Can you work these out from the model? Positions are in its coordinate system, mm. Face numbers are marked on the shaded views. A direction names the side the tool comes from. Round coordinates to 2 decimals unless told otherwise and drop trailing zeros. Loops run counter-clockwise (first coordinate to the right, second up) from the corner with the lowest first, then second, coordinate; pieces in that order, holes last. Notation, with made-up numbers: (85, 81) -> (125, 81) arc R27 cw to (125, 102) -> close; hole circle Ø11 at (-4.5, 69). An arc over 180 degrees is marked (long way). Answer as a JSON object with one key per item and string values.
```python
from build123d import *

# Parameters (mm, degrees)
SKETCH1_W           = 32
SKETCH1_H           = 32
BOSS_EXTRUDE1_DEPTH = 30
FILLET1_R           = 6
SKETCH2_R           = 1.5
BOSS_EXTRUDE2_DEPTH = 2.8


with BuildPart() as part:
    # Sketch1 → Boss-Extrude1 (new body)
    with BuildSketch(Plane(origin=(24, 0, 0), x_dir=(0, 0, -1), z_dir=(1, 0, 0))):
        Rectangle(SKETCH1_W, SKETCH1_H)
    extrude(amount=BOSS_EXTRUDE1_DEPTH)

    # Fillet1
    fillet1_edges = [part.edges().sort_by_distance(p)[0] for p in [
        (54, 0, -16),
        (54, 16, 0),
        (54, 0, 16),
        (24, 16, 0),
        (24, 0, -16),
        (24, -16, 0),
        (24, 0, 16),
        (39, 16, 16),
        (39, 16, -16),
        (39, -16, -16),
        (39, -16, 16),
        (54, -16, 0),
    ]]
    fillet(fillet1_edges, radius=FILLET1_R)

    # Sketch2 → Boss-Extrude2 (add)
    with BuildSketch(Plane(origin=(21.2, 0, 0), x_dir=(0, 0, -1), z_dir=(1, 0, 0))):
        with Locations((-4, -4)):
            Circle(SKETCH2_R)
        with Locations((4, -4)):
            Circle(SKETCH2_R)
        with Locations((-4, 4)):
            Circle(SKETCH2_R)
        with Locations((4, 4)):
            Circle(SKETCH2_R)
    extrude(amount=BOSS_EXTRUDE2_DEPTH)


solid = part.part
```
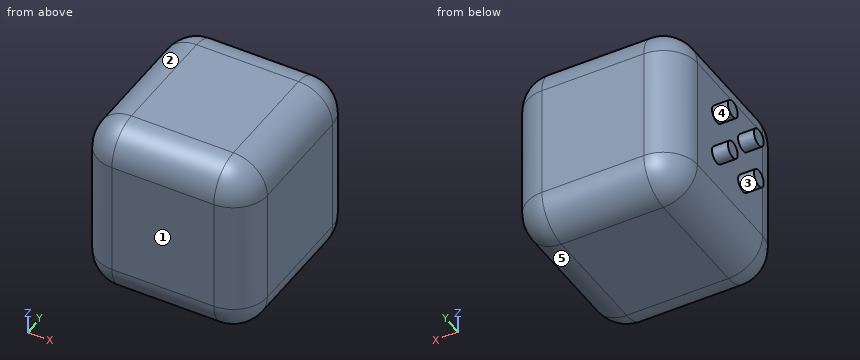
Q1. On a 3-axis mill with a long thin cutter (end or side, diameter ignored), from which of +Z, -Z, +X, -X, +Y, -Y can I reach the whole of each face in a straight line? I mean the marked faces 4 and 5. Say none if no direction works.
Determined:
{"face 4": "-X", "face 5": "-Z, +X, +Y, -Y"}
Q2. I want a section at D-D, the plane z = -9.5. Write out the boundary of the cut face in (x, y).
Determined:
{"outline": "(24, -10) arc R6 ccw to (30, -16) -> (48, -16) arc R6 ccw to (54, -10) -> (54, 10) arc R6 ccw to (48, 16) -> (30, 16) arc R6 ccw to (24, 10) -> close"}
Q3. I want a section at A-A, the plane y = 4. Write out the boundary of the cut face in (x, z), then the cut area to 3 significant figures.
Determined:
{"outline": "(21.2, -5.5) -> (24, -5.5) -> (24, -10) arc R6 ccw to (30, -16) -> (48, -16) arc R6 ccw to (54, -10) -> (54, 10) arc R6 ccw to (48, 16) -> (30, 16) arc R6 ccw to (24, 10) -> (24, 5.5) -> (21.2, 5.5) -> (21.2, 2.5) -> (24, 2.5) -> (24, -2.5) -> (21.2, -2.5) -> close", "area": "946 mm²"}
Q4. If I drill on L1, parallel to X at y = 4, z = -1.5; L2, parallel to Y at x = 52.5, z = -3; L3, parallel to X at y = 14, z = 9, over which ranges is the centre line in solid material (lowest first)? Write a range as [from, to].
Determined:
{"L1": "[24, 54]", "L2": "[-13.97, 13.97]", "L3": "[25.53, 52.47]"}
Q5. We'd pull the mould along Y, two halves only. Please class the marked faces 1, 2 and 3: pulls with the +Y half, pulls with the -Y half, needs draft (parallel to the pull), parting line crosses it, or undercut.
Determined:
{"face 1": "pulls with the -Y half", "face 2": "needs draft", "face 3": "undercut"}
Q6. I want a section at B-B, the plane x = 45.5. Write out the boundary of the cut face in (y, z).
Determined:
{"outline": "(-16, -10) arc R6 ccw to (-10, -16) -> (10, -16) arc R6 ccw to (16, -10) -> (16, 10) arc R6 ccw to (10, 16) -> (-10, 16) arc R6 ccw to (-16, 10) -> close"}
Q7. I'm going to push flat-ended pins straight in: pin 1 (2 mm diameter, centred on y = 6.5, z = -2, fed in from -X); pin 2 (1 mm diameter, centred on x = 47, z = -12.5, fed in from +Y). Where does each tip first touch, or does it pass through?
Determined:
{"pin 1": "x = 24", "pin 2": "y = 15.66"}
